Could you check a few things on this model? Use its own coordinates, in mm. A direction names the side the tool comes from. Round coordinates to 2 decimals unless told otherwise and drop trailing zeros. Loops run counter-clockwise (first coordinate to the right, second up) from the corner with the lowest first, then second, coordinate; pieces in that order, holes last. Notation, with made-up numbers: (72, 16) - (76, 16) arc R15 cw to (76, 28) - close; hole circle Ø6 at (85.25, -30). An arc over 180 degrees is marked (long way). Use one line per item in the form item = value.
```python
from build123d import *

# Parameters (mm, degrees)
EXTRUDE_THIN1_DEPTH = 1016
FILLET1_R           = 1.27


with BuildPart() as part:
    # Sketch1 → Extrude-Thin1 (new body)
    with BuildSketch(Plane.XY):
        with BuildLine():
            Line((0, 0), (-4.079695, 0.998592))
            ThreePointArc((-4.079695, 0.998592), (-8.001144, 3.52729), (-9.525, 7.9375))
            Line((-9.525, 7.9375), (-11.90625, 7.9375))
            Line((-11.90625, 7.9375), (-11.90625, 53.975))
            ThreePointArc((-11.90625, 53.975), (-16.66875, 58.7375), (-11.906249, 63.5))
            ThreePointArc((-11.906249, 63.5), (-13.570529, 67.254051), (-16.484535, 70.147372))
            ThreePointArc((-16.484535, 70.147372), (-20.860175, 75.589972), (-21.43125, 82.55))
            Line((-21.43125, 82.55), (-25.4, 82.55))
            Line((-25.4, 82.55), (-25.4, 101.6))
            Line((-25.4, 101.6), (0, 101.6))
            Line((0, 101.6), (0, 100.33))
            Line((0, 100.33), (-24.13, 100.33))
            Line((-24.13, 100.33), (-24.13, 83.82))
            Line((-24.13, 83.82), (-19.728013, 83.82))
            ThreePointArc((-19.728013, 83.82), (-19.950403, 76.819407), (-15.771635, 71.198406))
            ThreePointArc((-15.771635, 71.198406), (-12.006284, 67.154926), (-10.374537, 61.876196))
            ThreePointArc((-10.374537, 61.876196), (-15.395826, 58.880375), (-10.63625, 55.484093))
            Line((-10.63625, 55.484093), (-10.63625, 9.2075))
            Line((-10.63625, 9.2075), (-8.116059, 9.2075))
            ThreePointArc((-8.116059, 9.2075), (-7.369003, 4.835362), (-3.777749, 2.232175))
            Line((-3.777749, 2.232175), (0.301946, 1.233584))
            Line((0.301946, 1.233584), (0, 0))
        make_face()
    extrude(amount=-EXTRUDE_THIN1_DEPTH)

    # Fillet1
    fillet1_edges = [part.edges().sort_by_distance(p)[0] for p in [
        (-19.728013, 83.82, -508),
        (-10.374537, 61.876196, -508),
        (-10.63625, 55.484093, -508),
        (-8.116059, 9.2075, -508),
        (-11.90625, 7.9375, -508),
        (-25.4, 82.55, -508),
        (-25.4, 101.6, -508),
    ]]
    fillet(fillet1_edges, radius=FILLET1_R)


solid = part.part
```
1. If we section it at A-A, the plane y = 23: Write out the boundary of the cut face in (x, z).
Solution:
outline = (-11.91, -1016) - (-10.64, -1016) - (-10.64, 0) - (-11.91, 0) - close
2. We'd pull the mould along Y, two halves only. Please class faces 1 (the face through (-24.13, 92, -501)), 2 (the face through (-12, 101.6, -501)), 3 (the face through (-11.906, 31, -501)): +Y half, -Y half, draft (parallel to the pull), parting line (faces both ways), or undercut.
Solution:
face_1 = undercut
face_2 = +Y half
face_3 = draft
3. For P1, Ø2, axis at y = 33.5, z = -424.5, coming from the -X side; P2, Ø3, axis at x = -14.5, z = -471, coming from the -Y side; P3, Ø1.4, axis at y = 101, z = -434, coming from the +X side; P4, Ø4, axis at x = -12.5, y = 34, coming from the +Z side, each with a flat end and sliding along its axis, tell me the tip position at first contact or that it passes through.
Solution:
P1 = -11.91
P2 = 54.1
P3 = 0
P4 = 0
4. Please list where these lines run through material, in increasing order: line 1 along Y through (x, z) = (-16.25, -452.5); line 2 along Y through (x, z) = (-15, -667); line 3 along X through (y, z) = (12.5, -618.5).
Solution:
line_1 = 56.78 to 60.69, 69.98 to 71.54, 100.33 to 101.6
line_2 = 55.12 to 57.12, 60.36 to 62.36, 68.94 to 70.63, 100.33 to 101.6
line_3 = -11.91 to -10.64
5. On a 3-axis mill with a long thin cutter (end or side, diameter ignored), from which of +Z, -Z, +X, -X, +Y, -Y can I reach the whole of each face in a straight line? I mean faces 4 (the face through (-10.636, 32, -501)), 5 (the face through (-11.5, 51, 0)). Say none if no direction works.
Solution:
face_4 = +Z, -Z, +X
face_5 = +Z, +X, -X, +Y, -Y
